Work out the finished part from the listing and answer in its coordinate system (mm). A direction names the side the tool comes from. Round coordinates to 2 decimals unless told otherwise and drop trailing zeros. Write each loop counter-clockwise with the first axis right and the second up, starting at its lowest first coordinate (ties: lowest second). Pieces come first, ordered by that corner, then holes. Notation, with made-up numbers: (58, 0.25) -> (114, 0.25) arc R21 cw to (114, 8.25) -> close; hole circle Ø9 at (-40, 53). An arc over 180 degrees is marked (long way). One line per item, written item: value.
```python
from build123d import *

# Parameters (mm, degrees)
SKETCH1_W                  = 180
SKETCH1_H                  = 100
BOSS_EXTRUDE2_DEPTH        = 70
CUT_EXTRUDE1_DEPTH         = 70
SKETCH3_R                  = 5
CUT_EXTRUDE2_DEPTH         = 70
SKETCH4_R                  = 5
CUT_EXTRUDE3_DEPTH         = 50
SKETCH5_R                  = 10
CUT_EXTRUDE4_DEPTH         = 106
SKETCH6_R                  = 15
CUT_EXTRUDE5_DEPTH         = 40
SKETCH8_R                  = 15
SKETCH8_R_2                = 12.5
BOSS_EXTRUDE3_DEPTH        = 40
SKETCH10_R                 = 12.5
BOSS_EXTRUDE4_DEPTH        = 65
F_25_0MM_DOWEL_HOLE2_D     = 25
F_25_0MM_DOWEL_HOLE2_DEPTH = 20
F_25_0MM_DOWEL_HOLE2_TIP   = 7.510757738
SKETCH12_R                 = 10
SKETCH12_R_2               = 12.5
CUT_EXTRUDE6_DEPTH         = 20
SKETCH13_R                 = 25
SKETCH13_R_2               = 12.5
BOSS_EXTRUDE5_DEPTH        = 40
SKETCH14_R                 = 20
SKETCH14_R_2               = 10
CUT_EXTRUDE7_DEPTH         = 20
BOSS_EXTRUDE10_DEPTH       = 30
BOSS_EXTRUDE13_DEPTH       = 30


with BuildPart() as part:
    # Sketch1 → Boss-Extrude2 (new body)
    with BuildSketch(Plane.XY):
        with Locations((90, 50)):
            Rectangle(SKETCH1_W, SKETCH1_H)
    extrude(amount=BOSS_EXTRUDE2_DEPTH)

    # Sketch2 → Cut-Extrude1 (cut)
    with BuildSketch(Plane.XY.offset(70)):
        with BuildLine():
            Line((50, 100), (0, 100))
            Line((0, 100), (0, 50))
            ThreePointArc((0, 50), (14.644660941, 85.355339059), (50, 100))
        make_face()
        with BuildLine():
            ThreePointArc((50, 0), (14.644660941, 14.644660941), (0, 50))
            Line((0, 50), (0, 0))
            Line((0, 0), (50, 0))
        make_face()
        with BuildLine():
            Line((180, 0), (180, 50))
            ThreePointArc((180, 50), (165.355339059, 14.644660941), (130, 0))
            Line((130, 0), (180, 0))
        make_face()
        with BuildLine():
            Line((180, 100), (130, 100))
            ThreePointArc((130, 100), (165.355339059, 85.355339059), (180, 50))
            Line((180, 50), (180, 100))
        make_face()
    extrude(amount=-CUT_EXTRUDE1_DEPTH, mode=Mode.SUBTRACT)

    # Sketch3 → Cut-Extrude2 (cut)
    with BuildSketch(Plane.XY.offset(70)):
        with Locations((10, 50)):
            Circle(SKETCH3_R)
    extrude(amount=-CUT_EXTRUDE2_DEPTH, mode=Mode.SUBTRACT)

    # Sketch4 → Cut-Extrude3 (cut)
    with BuildSketch(Plane.XY.offset(70)):
        with BuildLine():
            ThreePointArc((10, 20), (21.458980338, 50), (10, 80))
            ThreePointArc((10, 80), (0, 50), (10, 20))
        make_face()
        with Locations((10, 50)):
            Circle(SKETCH4_R, mode=Mode.SUBTRACT)
    extrude(amount=-CUT_EXTRUDE3_DEPTH, mode=Mode.SUBTRACT)

    # Sketch5 → Cut-Extrude4 (cut)
    with BuildSketch(Plane.XY.offset(70)):
        with Locations((50, 50)):
            Circle(SKETCH5_R)
    extrude(amount=-CUT_EXTRUDE4_DEPTH, mode=Mode.SUBTRACT)

    # Sketch6 → Cut-Extrude5 (cut)
    with BuildSketch(Plane.XY.offset(70)):
        with Locations((130, 50)):
            Circle(SKETCH6_R)
    extrude(amount=-CUT_EXTRUDE5_DEPTH, mode=Mode.SUBTRACT)

    # Sketch8 → Boss-Extrude3 (add)
    with BuildSketch(Plane.XY.offset(70)):
        with Locations((130, 50)):
            Circle(SKETCH8_R)
        with Locations((130, 50)):
            Circle(SKETCH8_R_2, mode=Mode.SUBTRACT)
    extrude(amount=-BOSS_EXTRUDE3_DEPTH)

    # Sketch10 → Boss-Extrude4 (add)
    with BuildSketch(Plane.XY.offset(70)):
        with Locations((130, 50)):
            Circle(SKETCH10_R)
    extrude(amount=-BOSS_EXTRUDE4_DEPTH)

    # Ø25.0mm Dowel Hole2
    with Locations(Plane(origin=(130, 50, 70), x_dir=(1, 0, 0), z_dir=(0, 0, 1))):
        with Locations((0, 0)):
            Hole(F_25_0MM_DOWEL_HOLE2_D / 2, depth=F_25_0MM_DOWEL_HOLE2_DEPTH)
            with Locations((0, 0, -(F_25_0MM_DOWEL_HOLE2_DEPTH + F_25_0MM_DOWEL_HOLE2_TIP / 2))):  # 118° drill point
                Cone(0, F_25_0MM_DOWEL_HOLE2_D / 2, F_25_0MM_DOWEL_HOLE2_TIP, mode=Mode.SUBTRACT)

    # Sketch12 → Cut-Extrude6 (cut)
    with BuildSketch(Plane.XY.offset(70)):
        with BuildLine():
            ThreePointArc((130, 10), (170, 50), (130, 90))
            Line((130, 90), (20, 90))
            ThreePointArc((20, 90), (14.644660941, 85.355339059), (10, 80))
            ThreePointArc((10, 80), (21.458980338, 50), (10, 20))
            ThreePointArc((10, 20), (14.644660941, 14.644660941), (20, 10))
            Line((20, 10), (130, 10))
        make_face()
        with Locations((50, 50)):
            Circle(SKETCH12_R, mode=Mode.SUBTRACT)
        with Locations((130, 50)):
            Circle(SKETCH12_R_2, mode=Mode.SUBTRACT)
    extrude(amount=-CUT_EXTRUDE6_DEPTH, mode=Mode.SUBTRACT)

    # Sketch13 → Boss-Extrude5 (add)
    with BuildSketch(Plane.XY.offset(50)):
        with Locations((130, 50)):
            Circle(SKETCH13_R)
        with Locations((130, 50)):
            Circle(SKETCH13_R_2, mode=Mode.SUBTRACT)
    extrude(amount=BOSS_EXTRUDE5_DEPTH)

    # Sketch14 → Cut-Extrude7 (cut)
    with BuildSketch(Plane.XY.offset(50)):
        with Locations((50, 50)):
            Circle(SKETCH14_R)
        with Locations((50, 50)):
            Circle(SKETCH14_R_2, mode=Mode.SUBTRACT)
    extrude(amount=-CUT_EXTRUDE7_DEPTH, mode=Mode.SUBTRACT)

    # Sketch15 → Boss-Extrude10 (add)
    with BuildSketch(Plane.XY.offset(50)):
        with BuildLine():
            Line((105.505102572, 45), (105.505102572, 55))
            ThreePointArc((105.505102572, 55), (105, 50), (105.505102572, 45))
        make_face()
        with BuildLine():
            ThreePointArc((105.505102572, 45), (105, 50), (105.505102572, 55))
            Line((105.505102572, 55), (80.505102572, 55))
            Line((80.505102572, 55), (80.505102572, 45))
            Line((80.505102572, 45), (105.505102572, 45))
        make_face()
    extrude(amount=BOSS_EXTRUDE10_DEPTH)

    # Sketch16 → Boss-Extrude13 (add)
    with BuildSketch(Plane.XY.offset(50)):
        with BuildLine():
            Line((169.686269666, 55), (154.494897428, 55))
            ThreePointArc((154.494897428, 55), (155, 50), (154.494897428, 45))
            Line((154.494897428, 45), (169.686269666, 45))
            ThreePointArc((169.686269666, 45), (169.921490369, 47.495083498), (170, 50))
            ThreePointArc((170, 50), (169.921490369, 52.504916502), (169.686269666, 55))
        make_face()
    extrude(amount=BOSS_EXTRUDE13_DEPTH)


solid = part.part
```
(1) Consider probe 1 along Y at (x, z) = (130, 62); probe 2 along Y at (x, z) = (130, 75.5); probe 3 along Y at (x, z) = (101, 53). Determine where each line is inside the solid, lowest interval first.
Reported:
probe 1: y = 0 to 10, 25 to 37.5, 62.5 to 75, 90 to 100
probe 2: y = 25 to 37.5, 62.5 to 75
probe 3: y = 0 to 10, 45 to 55, 90 to 100
(2) For a pull along X with two mould halves and no side action, classify faces 6 (the face through (156.15, 19.73, 60.14)), 7 (the face through (93, 55, 65)) as pulls with the +X half, pulls with the -X half, needs draft (parallel to the pull), parting line crosses it, or undercut.
Reported:
face 6: undercut
face 7: needs draft
(3) Find section A-A on x = 12. Give the vertices of the cut face in (y, z), plus the area to 3 significant figures.
Reported:
outline: (17.5, 0) -> (45.42, 0) -> (45.42, 20) -> (22.4, 20) -> (22.4, 50) -> (17.5, 50) -> close; (54.58, 0) -> (82.5, 0) -> (82.5, 50) -> (77.6, 50) -> (77.6, 20) -> (54.58, 20) -> close
area: 1,410 mm2
(4) Find section B-B on z = 40. Give the vertices of the cut face in (x, y).
Reported:
outline: (10, 20) arc R50 ccw to (50, 0) -> (130, 0) arc R50 ccw to (130, 100) -> (50, 100) arc R50 ccw to (10, 80) arc R45 cw to start; hole circle Ø40 at (50, 50)
(5) Flat-ended cylindrical pins translate along their axes: pin 1 Ø13 at (x, y) = (10, 50) entering from +Z; pin 2 Ø18 at (x, y) = (50, 50) entering from +Z; pin 3 Ø1 at (x, z) = (34.5, 66.5) entering from -Y; pin 4 Ø4 at (y, z) = (60.5, 48.5) entering from -X. Find the tip coordinate at first contact, or state that the pin passes through.
Reported:
pin 1: stops at z = 20
pin 2: passes through
pin 3: stops at y = 2.3
pin 4: stops at x = 19.69
(6) Find section C-C on x = 91. Give the vertices of the cut face in (y, z), plus the area to 3 significant figures.
Reported:
outline: (0, 0) -> (100, 0) -> (100, 70) -> (90, 70) -> (90, 50) -> (55, 50) -> (55, 80) -> (45, 80) -> (45, 50) -> (10, 50) -> (10, 70) -> (0, 70) -> close
area: 5,700 mm2
(7) A tool of negligible diameter and unlimited length cuts with its end or side. For faces 1 (the face through (124.1, 61.5, 90)), 2 (the face through (100, 9, 70)), 3 (the face through (47.83, 40.24, 15.21)), 4 (the face through (153.846, 57.509, 69.72)), 5 (the face through (76, 90, 60)), from which of +Z, -Z, +X, -X, +Y, -Y can it reach the whole face along a straight path? Write none if from no direction.
Reported:
face 1: +Z, +X, -X, +Y, -Y
face 2: +Z, +X
face 3: +Z, -Z
face 4: +Z
face 5: +Z, -X
(8) Find section D-D on y = 22. Give the vertices of the cut face in (x, z), plus the area to 3 significant figures.
Reported:
outline: (8.58, 0) -> (171.42, 0) -> (171.42, 70) -> (158.57, 70) -> (158.57, 50) -> (11.69, 50) -> (11.69, 20) -> (8.58, 20) -> close
area: 8,310 mm2
